Source: three-view drawing plus pictorial views. Frame: mm from the lowest corner of the part. Round coordinates to 2 decimals unless told otherwise and drop trailing zeros. Loops run counter-clockwise (first coordinate to the right, second up) from the corner with the lowest first, then second, coordinate; pieces in that order, holes last. Notation, with made-up numbers: M 14,86 L 29,86 A35 cw 29,124 Z; hole C 39.25,18 d11. An arc over 180 degrees is marked long. Return JSON: item names as keys, results as strings. Group by question number.
1) Section D-D (z = 1.1). Count the separate pieces of the cut face and the enclosed holes in it, plus the area to 4 significant figures.
2) Section B-B (x = 31). Output: boundary loops of the cut face in (y, z), plus the area to 3 significant figures.
3) Contact query for flat-ended pins moving along their axis: P1, Ø1.5, axis at y = 2, z = 1.5, coming from the +X side; P2, Ø1.5, axis at x = 36.5, z = 2, coming from the -Y side; P3, Ø1.5, axis at y = 15, z = 1.5, coming from the -X side. Output: stop coordinate, or through.
4) Material intervals for line 1 (X direction, y = 21, z = 2.05); line 2 (X direction, y = 4, z = 1.5); line 3 (Y direction, x = 22, z = 0.95), sorted ascending. Write a range as from..to.
5) Section A-A (x = 103.5). Output: boundary loops of the cut face in (y, z), plus the area to 3 significant figures.
6) Section C-C (y = 12.5). Output: boundary loops of the cut face in (x, z), plus the area to 3 significant figures.
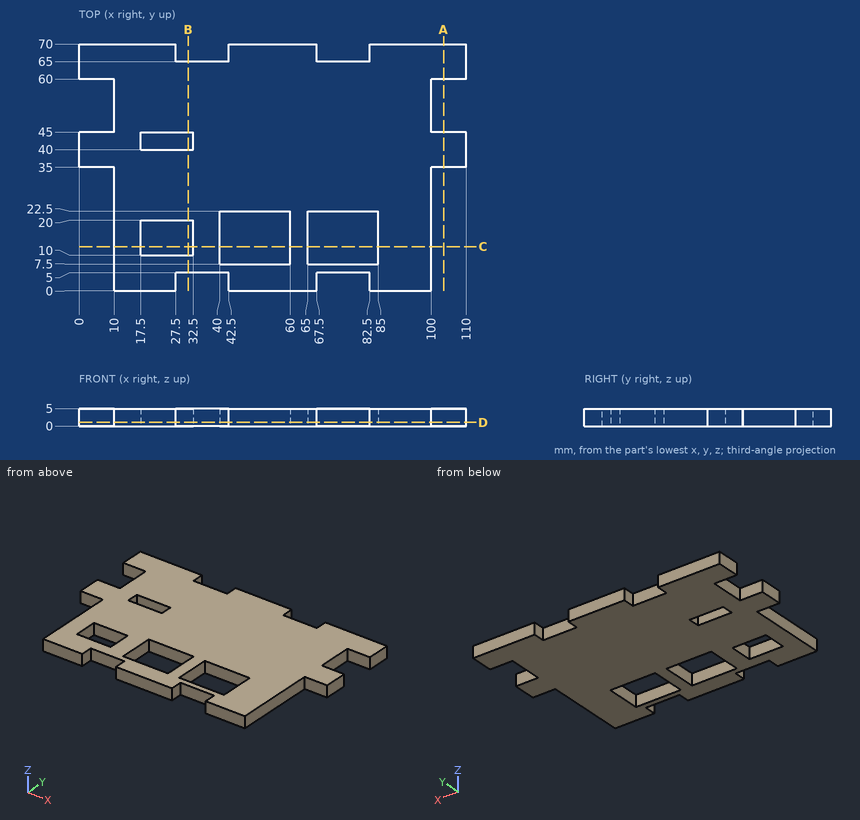
Returned:
{
 "1": {"separate pieces": "1", "enclosed holes": "4", "area": "5,575 mm^2"},
 "2": {"outline": "M 5,0 L 10,0 L 10,5 L 5,5 Z; M 20,0 L 40,0 L 40,5 L 20,5 Z; M 45,0 L 65,0 L 65,5 L 45,5 Z", "area": "225 mm^2"},
 "3": {"P1": "stops at x = 100", "P2": "stops at y = 5", "P3": "stops at x = 10"},
 "4": {"line 1": "x = 10..40, 60..65, 85..100", "line 2": "x = 10..27.5, 42.5..67.5, 82.5..100", "line 3": "y = 0..10, 20..40, 45..70"},
 "5": {"outline": "M 35,0 L 45,0 L 45,5 L 35,5 Z; M 60,0 L 70,0 L 70,5 L 60,5 Z", "area": "100 mm^2"},
 "6": {"outline": "M 10,0 L 17.5,0 L 17.5,5 L 10,5 Z; M 32.5,0 L 40,0 L 40,5 L 32.5,5 Z; M 60,0 L 65,0 L 65,5 L 60,5 Z; M 85,0 L 100,0 L 100,5 L 85,5 Z", "area": "175 mm^2"}
}
